Read the model definition and answer for the solid it produces. Units are mm, in the model's axes. Face numbers are marked on the shaded views. A direction names the side the tool comes from. Round coordinates to 2 decimals unless told otherwise and drop trailing zeros. Write each loop counter-clockwise with the first axis right and the second up, starting at its lowest first coordinate (ties: lowest second). Pieces come first, ordered by that corner, then holes. Notation, with made-up numbers: (-19, 29) - (3, 29) arc R20 cw to (3, 68) - close; hole circle Ø6 at (83, 1.5). An arc over 180 degrees is marked (long way). Use one line per item in the form item = value. Start each with the question number.
1) Consider line 1 along Z through (x, y) = (4, 0.5); line 2 along X through (y, z) = (13, 36); line 3 along X through (y, z) = (22, 12). Determine where each line is inside the solid, lowest interval first. Write a range as from..to.
2) Each of these flat-tipped pins is pushed along its axis until it touches: pin 1 (1.5 mm diameter, centred on x = -3, y = 7, fed in from +Z); pin 2 (1.5 mm diameter, centred on x = -2.5, z = 10.5, fed in from -Y); pin 3 (0.5 mm diameter, centred on x = -2.5, y = -10, fed in from +Z). Where does it stop, or does it pass through?
3) The part is cut by section B-B, the plane z = 16. Give the vertices of the cut face in (x, y).
4) For the marked faces 1 and 2, determine the directions among +Z, -Z, +X, -X, +Y, -Y from which every point of the face is accessible in a straight line to the end or side of a thin tool.
5) The part is cut by section D-D, the plane z = 22. Give the vertices of the cut face in (x, y).
6) The part is cut by section C-C, the plane x = 4. Give the vertices of the cut face in (y, z), plus the area to 3 significant figures.
7) The part is cut by section A-A, the plane y = 9. Give the vertices of the cut face in (x, z).
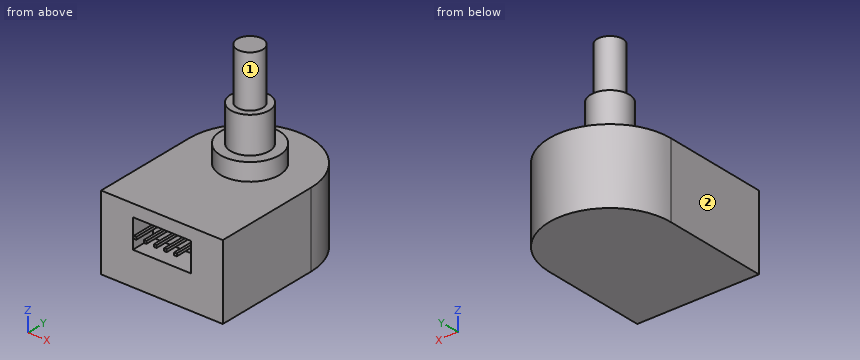
from build123d import *

# Parameters (mm, degrees)
BOSS_EXTRU_1_DEPTH      = 18.3
ESQUISSE2_R             = 7.25
BOSS_EXTRU_2_DEPTH      = 4.3
ESQUISSE3_R             = 4.7625
BOSS_EXTRU_3_DEPTH      = 8.9
ESQUISSE4_R             = 3.175
BOSS_EXTRU_4_DEPTH      = 12.7
ESQUISSE5_W             = 14.36
ESQUISSE5_H             = 7.1
ENL_V_MAT_EXTRU_2_DEPTH = 6
ESQUISSE6_W             = 0.64
ESQUISSE6_H             = 0.64
BOSS_EXTRU_5_DEPTH      = 8


with BuildPart() as part:
    # Esquisse1 → Boss.-Extru.1 (new body)
    with BuildSketch(Plane.XY):
        with BuildLine():
            Line((-15, -13.1), (15, -13.1))
            Line((15, -13.1), (15, 13.1))
            ThreePointArc((15, 13.1), (0, 28.1), (-15, 13.1))
            Line((-15, 13.1), (-15, -13.1))
        make_face()
    extrude(amount=BOSS_EXTRU_1_DEPTH)

    # Esquisse2 → Boss.-Extru.2 (add)
    with BuildSketch(Plane.XY.offset(18.3)):
        with Locations((0, 13.1)):
            Circle(ESQUISSE2_R)
    extrude(amount=BOSS_EXTRU_2_DEPTH)

    # Esquisse3 → Boss.-Extru.3 (add)
    with BuildSketch(Plane.XY.offset(22.6)):
        with Locations((0, 13.1)):
            Circle(ESQUISSE3_R)
    extrude(amount=BOSS_EXTRU_3_DEPTH)

    # Esquisse4 → Boss.-Extru.4 (add)
    with BuildSketch(Plane.XY.offset(31.5)):
        with Locations((0, 13.1)):
            Circle(ESQUISSE4_R)
    extrude(amount=BOSS_EXTRU_4_DEPTH)

    # Esquisse5 → Enlèv. mat.-Extru.2 (cut)
    with BuildSketch(Plane.XZ.offset(13.1)):
        with Locations((0, 11.75)):
            Rectangle(ESQUISSE5_W, ESQUISSE5_H)
    extrude(amount=-ENL_V_MAT_EXTRU_2_DEPTH, mode=Mode.SUBTRACT)

    # Esquisse6 → Boss.-Extru.5 (add)
    with BuildSketch(Plane.XZ.offset(7.1)):
        with Locations((-5, 12.457086597)):
            Rectangle(ESQUISSE6_W, ESQUISSE6_H)
        with Locations((-2.5, 12.457086597)):
            Rectangle(ESQUISSE6_W, ESQUISSE6_H)
        with Locations((0, 12.457086597)):
            Rectangle(ESQUISSE6_W, ESQUISSE6_H)
        with Locations((2.5, 12.457086597)):
            Rectangle(ESQUISSE6_W, ESQUISSE6_H)
        with Locations((5, 12.457086597)):
            Rectangle(ESQUISSE6_W, ESQUISSE6_H)
    extrude(amount=BOSS_EXTRU_5_DEPTH)


solid = part.part
Geometry results:
q1.line_1 = 0..18.3
q1.line_2 = -3.17..3.17
q1.line_3 = -12.07..12.07
q2.pin_1 = 22.6
q2.pin_2 = -7.1
q2.pin_3 = 18.3
q3.outline = (-15, -13.1) - (15, -13.1) - (15, 13.1) arc R15 ccw to (-15, 13.1) - close
q4.face_1 = +Z
q4.face_2 = +Z, -Z, -X, +Y, -Y
q5.outline = circle Ø14.5 at (0, 13.1)
q6.outline = (-13.1, 0) - (27.56, 0) - (27.56, 18.3) - (19.15, 18.3) - (19.15, 22.6) - (15.68, 22.6) - (15.68, 31.5) - (10.52, 31.5) - (10.52, 22.6) - (7.05, 22.6) - (7.05, 18.3) - (-13.1, 18.3) - (-13.1, 15.3) - (-7.1, 15.3) - (-7.1, 8.2) - (-13.1, 8.2) - close
q6.area = 799 mm2
q7.outline = (-15, 0) - (15, 0) - (15, 18.3) - (5.98, 18.3) - (5.98, 22.6) - (2.42, 22.6) - (2.42, 31.5) - (-2.42, 31.5) - (-2.42, 22.6) - (-5.98, 22.6) - (-5.98, 18.3) - (-15, 18.3) - close
